Verification items for the finished model (mm, model axes). Face numbers are marked on the shaded views. Coordinates: 2 decimals unless noted, no trailing zeros. Order: outer loops, then holes, each group sorted by start corner. A loop starts at its lowest first (then second) coordinate and runs counter-clockwise, first axis right, second up. Notation, with made-up numbers: (-35, 0) -> (0, 0) arc R30 ccw to (0, 28) -> close; hole circle Ø6 at (38, 45.25). An arc over 180 degrees is marked (long way). Write item = value, one per line. Start each with the question number.
1. Go/stop test with flat-tipped pins: P1, Ø8.5, axis at y = -1.5, z = -4.5, coming from the +X side; P2, Ø1.2, axis at x = 1.5, z = -18, coming from the +Y side; P3, Ø5, axis at x = -2, y = 0.5, coming from the +Z side. Record where each tip stops, or that it passes through.
2. Release check for a two-part mould opening along X. For the marked faces 1, 2, 3 and 4 record: +X half, -X half, draft (parallel to the pull), parting line (faces both ways), or undercut.
3. Cross-section at C-C on y = -7.25. Record the cut outline in (x, z).
4. Cross-section at A-A on z = 0. Record the cut outline in (x, y).
5. Cross-section at D-D on y = 0. Record the cut outline in (x, z), plus the area to 3 significant figures.
6. Cross-section at B-B on x = 6.25. Record the cut outline in (y, z).
7. Thickness scan on line 1 along X through (y, z) = (-2.25, 14); line 2 along Z through (x, y) = (-6.6, 0); line 3 along Y through (x, z) = (-5.55, 0). Record the ranges inside material, lowest first. Write a range as from..to.
from build123d import *

# Parameters (mm, degrees)
BOSS_EXTRUDE1_DEPTH     = 13.97
SKETCH5_R               = 1
BOSS_EXTRUDE4_DEPTH     = 2.5
SKETCH6_W               = 10
SKETCH6_H               = 8.89
CUT_EXTRUDE1_DEPTH      = 2.5
FILLET1_R               = 7.5
SKETCH4_R               = 3.1877
CUT_EXTRUDE2_DEPTH      = 13.5
CUT_EXTRUDE2_DEPTH_BACK = 6


with BuildPart() as part:
    # Sketch1 → Boss-Extrude1 (new body, symmetric)
    with BuildSketch(Plane(origin=(0, 0, 0), x_dir=(1, 0, 0), z_dir=(0, 1, 0))):
        Polygon((-7.5, -17.5), (-7.5, 20), (7.5, 20), (7.5, -17.5), (5, -17.5), (5, 17.5), (-5, 17.5), (-5, -17.5), align=None)
    extrude(amount=BOSS_EXTRUDE1_DEPTH, both=True)

    # Sketch5 → Boss-Extrude4 (add)
    with BuildSketch(Plane(origin=(7.5, 0, 0), x_dir=(0, 0, -1), z_dir=(1, 0, 0))):
        with Locations((-12.5, 0)):
            Circle(SKETCH5_R)
    extrude(amount=BOSS_EXTRUDE4_DEPTH)

    # Sketch6 → Cut-Extrude1 (cut)
    with BuildSketch(Plane(origin=(0, 0, -20), x_dir=(-1, 0, 0), z_dir=(0, 0, -1))):
        with Locations((0, -9.525)):
            Rectangle(SKETCH6_W, SKETCH6_H)
    cut_extrude1 = extrude(amount=-CUT_EXTRUDE1_DEPTH, mode=Mode.SUBTRACT)

    # Fillet1
    fillet1_edges = [part.edges().sort_by_distance(p)[0] for p in [
        (6.25, -13.97, 17.5),
        (-6.25, 13.97, 17.5),
        (6.25, 13.97, 17.5),
        (-6.25, -13.97, 17.5),
    ]]
    fillet(fillet1_edges, radius=FILLET1_R)

    # Sketch4 → Cut-Extrude2 (cut, two sides)
    with BuildSketch(Plane.ZY.offset(-5)) as cut_extrude2_sk:
        Circle(SKETCH4_R)
    extrude(amount=CUT_EXTRUDE2_DEPTH, mode=Mode.SUBTRACT)
    extrude(cut_extrude2_sk.sketch, amount=-CUT_EXTRUDE2_DEPTH_BACK, mode=Mode.SUBTRACT)

    # Mirror2: Cut-Extrude1 across plane
    add(cut_extrude1.mirror(Plane.ZX), mode=Mode.SUBTRACT)


solid = part.part
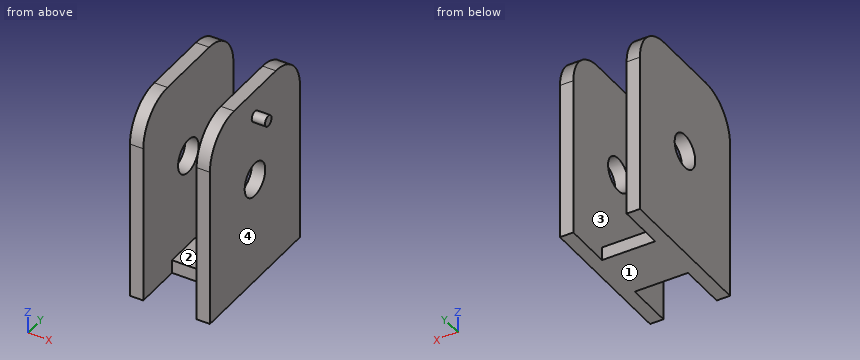
Worked out:
q1.P1 = 7.5
q1.P2 = 5.08
q1.P3 = -17.5
q2.face_1 = draft
q2.face_2 = undercut
q2.face_3 = undercut
q2.face_4 = +X half
q3.outline = (-7.5, -20) -> (-5, -20) -> (-5, 17.46) -> (-7.5, 17.46) -> close; (5, -20) -> (7.5, -20) -> (7.5, 17.46) -> (5, 17.46) -> close
q4.outline = (-7.5, -13.97) -> (-5, -13.97) -> (-5, -3.19) -> (-7.5, -3.19) -> close; (-7.5, 3.19) -> (-5, 3.19) -> (-5, 13.97) -> (-7.5, 13.97) -> close; (5, -13.97) -> (7.5, -13.97) -> (7.5, -3.19) -> (5, -3.19) -> close; (5, 3.19) -> (7.5, 3.19) -> (7.5, 13.97) -> (5, 13.97) -> close
q5.outline = (-7.5, -20) -> (7.5, -20) -> (7.5, -3.19) -> (5, -3.19) -> (5, -17.5) -> (-5, -17.5) -> (-5, -3.19) -> (-7.5, -3.19) -> close; (-7.5, 3.19) -> (-5, 3.19) -> (-5, 17.5) -> (-7.5, 17.5) -> close; (5, 3.19) -> (7.5, 3.19) -> (7.5, 11.5) -> (10, 11.5) -> (10, 13.5) -> (7.5, 13.5) -> (7.5, 17.5) -> (5, 17.5) -> close
q5.area = 186 mm²
q6.outline = (-13.97, -20) -> (13.97, -20) -> (13.97, 10) arc R7.5 ccw to (6.47, 17.5) -> (-6.47, 17.5) arc R7.5 ccw to (-13.97, 10) -> close; hole circle Ø6.38 at (0, 0)
q7.line_1 = -7.5..-5, 5..7.5
q7.line_2 = -20..-3.19, 3.19..17.5
q7.line_3 = -13.97..-3.19, 3.19..13.97
